The listing builds one solid part. Answer for the finished solid, in the listing's coordinates (mm). Give positions to 0.01 mm unless a question says otherwise; leave off trailing zeros. Order: outer loops, then holes, each group sorted by start corner. A loop starts at its lowest first (then second) coordinate and runs counter-clockwise, first axis right, second up.
Autodesk Inventor part; units mm, degrees
ref_plane "YZ Plane" through (0, 0, 0) normal (1, 0, 0) x (0, 1, 0)
ref_plane "XZ Plane" through (0, 0, 0) normal (0, 1, 0) x (-1, 0, 0)
ref_plane "XY Plane" through (0, 0, 0) normal (0, 0, 1) x (1, 0, 0)
ref_plane "Work Plane2" through (35.545, -31.609, 1.6) normal (0, 0, 1) x (1, 0, 0)
sketch "Sketch2" plane through (35.545, -31.609, 1.6) normal (0, 0, 1) x (1, 0, 0)
  line L0 (-4.7778, 3.1171) -> (341.5466, 3.1925) construction
  line L1 (341.5466, 3.1925) -> (341.5765, -133.848) construction
  line L2 (341.5765, -133.848) -> (-4.7479, -133.9235) construction
  line L3 (-4.7479, -133.9235) -> (-4.7778, 3.1171) construction
  point P0 (-35.545, 31.609)
ref_plane "Work Plane1" through (371.545, -162.609, 0) normal (0, 0, -1) x (-1, 0, 0)
sketch "Sketch9" plane through (371.545, -162.609, 0) normal (0, 0, -1) x (-1, 0, 0)
  line L0 (336, 131) -> (0, 131)
  line L1 (-2, 129) -> (-2, 2)
  line L2 (-1.9796, 129.2846) -> (-2, 129)
  line L3 (-1.919, 129.5635) -> (-1.9796, 129.2846)
  line L4 (-1.8193, 129.8308) -> (-1.919, 129.5635)
  line L5 (-1.6825, 130.0813) -> (-1.8193, 129.8308)
  line L6 (-1.5115, 130.3097) -> (-1.6825, 130.0813)
  line L7 (-1.3097, 130.5115) -> (-1.5115, 130.3097)
  line L8 (-1.0813, 130.6825) -> (-1.3097, 130.5115)
  line L9 (-0.8308, 130.8193) -> (-1.0813, 130.6825)
  line L10 (-0.5635, 130.919) -> (-0.8308, 130.8193)
  line L11 (-0.2846, 130.9796) -> (-0.5635, 130.919)
  line L12 (0, 131) -> (-0.2846, 130.9796)
  circle A0 centre (2.362, 128.645) radius 1.1
  circle A1 centre (68.695, 128.645) radius 1.1
  circle A2 centre (135.028, 128.645) radius 1.1
  circle A3 centre (201.361, 128.645) radius 1.1
  circle A4 centre (267.694, 128.645) radius 1.1
  circle A5 centre (334.027, 128.645) radius 1.1
  line L13 (338, 2) -> (338, 129)
  line L14 (338, 129) -> (337.9796, 129.2846)
  line L15 (337.9796, 129.2846) -> (337.919, 129.5635)
  line L16 (337.919, 129.5635) -> (337.8193, 129.8308)
  line L17 (337.8193, 129.8308) -> (337.6825, 130.0813)
  line L18 (337.6825, 130.0813) -> (337.5115, 130.3097)
  line L19 (337.5115, 130.3097) -> (337.3097, 130.5115)
  line L20 (337.3097, 130.5115) -> (337.0813, 130.6825)
  line L21 (337.0813, 130.6825) -> (336.8308, 130.8193)
  line L22 (336.8308, 130.8193) -> (336.5635, 130.919)
  line L23 (336.5635, 130.919) -> (336.2846, 130.9796)
  line L24 (336.2846, 130.9796) -> (336, 131)
  line L25 (0, 0) -> (336, 0)
  line L26 (336, 0) -> (336.2846, 0.0204)
  line L27 (336.2846, 0.0204) -> (336.5635, 0.081)
  line L28 (336.5635, 0.081) -> (336.8308, 0.1807)
  line L29 (336.8308, 0.1807) -> (337.0813, 0.3175)
  line L30 (337.0813, 0.3175) -> (337.3097, 0.4885)
  line L31 (337.3097, 0.4885) -> (337.5115, 0.6903)
  line L32 (337.5115, 0.6903) -> (337.6825, 0.9187)
  line L33 (337.6825, 0.9187) -> (337.8193, 1.1692)
  line L34 (337.8193, 1.1692) -> (337.919, 1.4365)
  line L35 (337.919, 1.4365) -> (337.9796, 1.7154)
  line L36 (337.9796, 1.7154) -> (338, 2)
  circle A6 centre (334.02, 2.37) radius 1.1
  circle A7 centre (267.687, 2.37) radius 1.1
  circle A8 centre (201.354, 2.37) radius 1.1
  circle A9 centre (135.021, 2.37) radius 1.1
  circle A10 centre (68.688, 2.37) radius 1.1
  circle A11 centre (2.355, 2.37) radius 1.1
  line L37 (-0.2846, 0.0204) -> (0, 0)
  line L38 (-0.5635, 0.081) -> (-0.2846, 0.0204)
  line L39 (-0.8308, 0.1807) -> (-0.5635, 0.081)
  line L40 (-1.0813, 0.3175) -> (-0.8308, 0.1807)
  line L41 (-1.3097, 0.4885) -> (-1.0813, 0.3175)
  line L42 (-1.5115, 0.6903) -> (-1.3097, 0.4885)
  line L43 (-1.6825, 0.9187) -> (-1.5115, 0.6903)
  line L44 (-1.8193, 1.1692) -> (-1.6825, 0.9187)
  line L45 (-1.919, 1.4365) -> (-1.8193, 1.1692)
  line L46 (-1.9796, 1.7154) -> (-1.919, 1.4365)
  line L47 (-2, 2) -> (-1.9796, 1.7154)
  circle A12 centre (41.979, 103.44) radius 1.1
  circle A13 centre (125.979, 103.44) radius 1.1
  circle A14 centre (210.039, 103.527) radius 1.1
  circle A15 centre (294.039, 103.527) radius 1.1
  point P0 (371.545, 162.609)
ref_plane "Work Plane3" through (371.545, -162.609, 0) normal (0, 0, 1) x (1, 0, 0)
sketch "Sketch10" plane through (371.545, -162.609, 0) normal (0, 0, 1) x (1, 0, 0)
  circle A0 centre (-294.039, 103.527) radius 1.1
  circle A1 centre (-210.039, 103.527) radius 1.1
  circle A2 centre (-125.979, 103.44) radius 1.1
  circle A3 centre (-41.979, 103.44) radius 1.1
  line L0 (-294.039, 113.527) -> (-41.979, 113.527)
  line L1 (-31.979, 103.527) -> (-31.979, 103.527)
  line L2 (-41.979, 93.527) -> (-294.039, 93.527)
  line L3 (-304.039, 103.527) -> (-304.039, 103.527)
  arc A4 (-31.979, 103.527) -> (-41.979, 113.527) centre (-41.979, 103.527) ccw
  arc A5 (-41.979, 93.527) -> (-31.979, 103.527) centre (-41.979, 103.527) ccw
  arc A6 (-294.039, 113.527) -> (-304.039, 103.527) centre (-294.039, 103.527) ccw
  arc A7 (-304.039, 103.527) -> (-294.039, 93.527) centre (-294.039, 103.527) ccw
  point P0 (-371.545, 162.609)
  point P1 (-31.979, 103.527)
  dimension "d89" = 10
  dimension "d90" = 10
  dimension "d91" = 10
  dimension "d92" = 10
  dimension "d93" = 10
extrude "Extrusion4" add sketch "Sketch10" along normal blind 3
properties part number "foot4"
1) Find section B-B (y = -53). Write down the section's boundary in (x, z).
Geometry says:
outline: (69.57, 0) - (337.5, 0) - (337.5, 3) - (69.57, 3) - close
2) Straight lines are drawn through the part: probe 1 along X at (y, z) = (-59, 2.85); probe 2 along X at (y, z) = (-58.75, 2.1); probe 3 along X at (y, z) = (-51, 1.75). For each, find the intervals that lie inside material, in ascending order.
Geometry says:
probe 1: x = 67.51 to 76.41, 78.6 to 160.41, 162.6 to 244.48, 246.65 to 328.48, 330.65 to 339.57
probe 2: x = 67.51 to 76.46, 78.55 to 160.46, 162.55 to 244.55, 246.58 to 328.55, 330.58 to 339.56
probe 3: x = 71.62 to 335.46
3) Find section C-C (y = -66.5). Write down the section's boundary in (x, z), then the cut area to 3 significant figures.
Geometry says:
outline: (70.8, 0) - (336.27, 0) - (336.27, 3) - (70.8, 3) - close
area: 796 mm2
4) Given P1, Ø3.5, axis at x = 245.566, y = -59.169, coming from the +Z side, flat-ended and moving along its own axis, determine where the tip first touches the part or whether it passes through.
Geometry says:
P1: stops at z = 3
5) Find section A-A (z = 1.1). Write down the section's boundary in (x, y), then the cut area to 3 significant figures.
Geometry says:
outline: (77.51, -69.08) - (329.57, -69.08) arc R10 ccw to (329.57, -49.08) - (77.51, -49.08) arc R10 ccw to start; hole circle Ø2.2 at (77.51, -59.08); hole circle Ø2.2 at (161.51, -59.08); hole circle Ø2.2 at (245.57, -59.17); hole circle Ø2.2 at (329.57, -59.17)
area: 5,340 mm2
